Input: part model. Units: mm. Frame: model coordinates. A direction names the side the tool comes from. Give positions to 0.01 mm unless a question says otherwise; leave off trailing zeros. Loops run counter-clockwise (first coordinate to the right, second up) from the corner with the lowest first, then second, coordinate; pieces in that order, holes last. Notation, with made-up numbers: M 65.25,8.5 L 111.25,8.5 A9 cw 111.25,24.5 Z; hole C -31.5,49.25 d7. An arc over 180 degrees is marked long. Answer as a JSON object with one key per item and string values. Group by question number.
1) Draft query along Y for faces 1 (the cylindrical face through (416.743, 537.928, 2.884)), 2 (the cylindrical face through (417.415, 544.716, 2.884)), 3 (the cylindrical face through (416.547, 551.546, 2.884)). Return one class per face: +Y half, -Y half, draft (parallel to the pull), parting line (faces both ways), or undercut.
2) Section query D-D on y = 552. Return loops of the section in (x, z), plus the area to 3 significant figures.
3) Access query for faces 4 (the flat face through (404, 549, 0)), 5 (the flat face through (400, 553.789, 3)). Directions: +Z, -Z, +X, -X, +Y, -Y. A direction counts if a zero-diameter tool reaches every point of the face in a straight line with its end or side. Return the directions, or none.
4) Section query C-C on x = 426. Return loops of the section in (y, z), plus the area to 3 significant figures.
5) Section query A-A on x = 408. Return loops of the section in (y, z).
6) First-contact query: P1, Ø1.3, axis at y = 552.5, z = 3, coming from the +X side; P2, Ø3, axis at y = 556, z = 3, coming from the -X side; P3, Ø1, axis at x = 420, z = 1.5, coming from the -Y side; P4, Ø1, axis at x = 396, y = 543.5, coming from the -Z side. Flat tips, straight axial feed; report the tip coordinate or a pass-through.
7) Section query B-B on y = 556. Return loops of the section in (x, z), plus the area to 3 significant figures.
8) Ray query, L1, parallel to Y at x = 397, z = 4.4; L2, parallel to Y at x = 403.5, z = 5.4; L3, parallel to X at y = 556, z = 3.55. Return the intervals inside material, ascending.
from build123d import *

# Parameters (mm, degrees)
SKETCH1_R           = 1.45
SKETCH1_W           = 3.400011
SKETCH1_H           = 6.1
BOSS_EXTRUDE2_DEPTH = 5.85


with BuildPart() as part:
    # Sketch1 → Boss-Extrude2 (new body)
    with BuildSketch(Plane.XY):
        with BuildLine():
            Line((388.472923735, 562.888903138), (410.424633118, 562.888903138))
            ThreePointArc((410.424633118, 562.888903138), (412.211329852, 562.148829119), (412.95140387, 560.362132386))
            ThreePointArc((412.95140387, 560.362132386), (416.644097047, 551.447182437), (425.559046996, 547.75448926))
            ThreePointArc((425.559046996, 547.75448926), (428.674633119, 544.638903138), (425.559046996, 541.523317015))
            ThreePointArc((425.559046996, 541.523317015), (416.644097047, 537.830623838), (412.95140387, 528.915673889))
            ThreePointArc((412.95140387, 528.915673889), (412.50422307, 527.836083937), (411.424633118, 527.388903138))
            Line((411.424633118, 527.388903138), (389.472923735, 527.388903138))
            add(Edge.make_bspline(
                [(387.555122745, 529.304742909), (387.449571593, 527.388903138), (389.472923735, 527.388903138)],
                knots=[0, 0, 0, 1, 1, 1], degree=2))
            Line((387.555122745, 529.304742909), (387.555122745, 561.972040272))
            add(Edge.make_bspline(
                [(387.555122745, 561.972040272), (387.504608679, 562.888903138), (388.472923735, 562.888903138)],
                knots=[0, 0, 0, 1, 1, 1], degree=2))
        make_face()
        with Locations((425.559046996, 544.638903138)):
            Circle(SKETCH1_R, mode=Mode.SUBTRACT)
        with Locations((399.559046996, 532.438903138)):
            Circle(SKETCH1_R, mode=Mode.SUBTRACT)
        Polygon((405.566920996, 551.188903138), (405.566920996, 553.788903138), (408.562971247, 553.788903138), (408.562971247, 559.888903138), (402.762971247, 559.888903138), (402.762971247, 553.788903138), (396.355122745, 553.788903138), (396.355122745, 559.888903138), (390.555122745, 559.888903138), (390.555122745, 553.788903138), (393.551172996, 553.788903138), (393.551172996, 551.188903138), align=None, mode=Mode.SUBTRACT)
        with Locations((394.409041496, 532.438903138)):
            Rectangle(SKETCH1_W, SKETCH1_H, mode=Mode.SUBTRACT)
        with Locations((404.709052496, 532.438903138)):
            Rectangle(SKETCH1_W, SKETCH1_H, mode=Mode.SUBTRACT)
        with BuildLine():
            Line((396.165690223, 548.138903138), (413.915690223, 548.138903138))
            ThreePointArc((413.915690223, 548.138903138), (417.415690223, 544.638903138), (413.915690223, 541.138903138))
            Line((413.915690223, 541.138903138), (396.165690223, 541.138903138))
            ThreePointArc((396.165690223, 541.138903138), (392.665690223, 544.638903138), (396.165690223, 548.138903138))
        make_face(mode=Mode.SUBTRACT)
    extrude(amount=BOSS_EXTRUDE2_DEPTH)


solid = part.part
Output:
{
 "1": {"face 1": "-Y half", "face 2": "undercut", "face 3": "+Y half"},
 "2": {"outline": "M 387.56,0 L 393.55,0 L 393.55,5.85 L 387.56,5.85 Z; M 405.57,0 L 416.12,0 L 416.12,5.85 L 405.57,5.85 Z", "area": "96.8 mm^2"},
 "3": {"face 4": "-Z, +X, -X, +Y, -Y", "face 5": "+Z, -Z"},
 "4": {"outline": "M 541.55,0 L 543.26,0 L 543.26,5.85 L 541.55,5.85 Z; M 546.02,0 L 547.72,0 L 547.72,5.85 L 546.02,5.85 Z", "area": "19.9 mm^2"},
 "5": {"outline": "M 527.39,0 L 541.14,0 L 541.14,5.85 L 527.39,5.85 Z; M 548.14,0 L 553.79,0 L 553.79,5.85 L 548.14,5.85 Z; M 559.89,0 L 562.89,0 L 562.89,5.85 L 559.89,5.85 Z"},
 "6": {"P1": "stops at x = 416.26", "P2": "stops at x = 387.56", "P3": "stops at y = 539.97", "P4": "passes through"},
 "7": {"outline": "M 387.56,0 L 390.56,0 L 390.56,5.85 L 387.56,5.85 Z; M 396.36,0 L 402.76,0 L 402.76,5.85 L 396.36,5.85 Z; M 408.56,0 L 413.73,0 L 413.73,5.85 L 408.56,5.85 Z", "area": "85.3 mm^2"},
 "8": {"L1": "y = 527.39 to 541.14, 548.14 to 551.19, 553.79 to 562.89", "L2": "y = 527.39 to 529.39, 535.49 to 541.14, 548.14 to 551.19, 559.89 to 562.89", "L3": "x = 387.56 to 390.56, 396.36 to 402.76, 408.56 to 413.73"}
}
